Autodesk Fusion 360 part; units mm, degrees
sketch "Sketch1" plane through (0, 0, 0) normal (0, 0, 1) x (1, 0, 0)
  line L0 (-400.05, 260.35) -> (-387.35, 273.05)
  line L1 (-400.05, 12.7) -> (-387.35, 0)
  line L2 (-400.05, 260.35) -> (-400.05, 12.7)
  line L3 (0, 260.35) -> (-12.7, 273.05)
  line L4 (0, 12.7) -> (-12.7, 0)
  line L5 (0, 260.35) -> (0, 12.7)
  line L6 (-387.35, 0) -> (-12.7, 0)
  line L7 (-387.35, 273.05) -> (-12.7, 273.05)
  line L8 (-6.35, 257.7197) -> (-15.3303, 266.7)
  line L9 (-384.7197, 266.7) -> (-15.3303, 266.7)
  line L10 (-393.7, 257.7197) -> (-384.7197, 266.7)
  line L11 (-393.7, 257.7197) -> (-393.7, 15.3303)
  line L12 (-393.7, 15.3303) -> (-384.7197, 6.35)
  line L13 (-384.7197, 6.35) -> (-15.3303, 6.35)
  line L14 (-6.35, 15.3303) -> (-15.3303, 6.35)
  line L15 (-6.35, 257.7197) -> (-6.35, 15.3303)
  dimension "d5" = 6.35
extrude "Extrude1" add sketch "Sketch1" along normal blind 0.254 contours L0 L1 L2 L3 L4 L5 L6 L7 | L8 L9 L10 L11 L12 L13 L14 L15
extrude "Extrude2" add sketch "Sketch1" along normal blind 69.85
sketch "Sketch2" plane through (0, 0, 69.85) normal (0, 0, 1) x (-1, 0, 0)
  line L0 (393.7, -15.3303) -> (393.7, -257.7197)
  line L1 (393.7, -257.7197) -> (384.7197, -266.7)
  line L2 (384.7197, -266.7) -> (15.3303, -266.7)
  line L3 (15.3303, -266.7) -> (6.35, -257.7197)
  line L4 (6.35, -257.7197) -> (6.35, -15.3303)
  line L5 (6.35, -15.3303) -> (15.3303, -6.35)
  line L6 (15.3303, -6.35) -> (384.7197, -6.35)
  line L7 (384.7197, -6.35) -> (393.7, -15.3303)
  line L8 (400.05, -260.35) -> (400.05, -12.7)
  line L9 (400.05, -12.7) -> (387.35, 0)
  line L10 (387.35, 0) -> (12.7, 0)
  line L11 (12.7, 0) -> (0, -12.7)
  line L12 (0, -12.7) -> (0, -260.35)
  line L13 (0, -260.35) -> (12.7, -273.05)
  line L14 (12.7, -273.05) -> (387.35, -273.05)
  line L15 (387.35, -273.05) -> (400.05, -260.35)
  line L16 (393.7, -162.4342) -> (393.7, -166.61)
  line L17 (295.275, -266.7) -> (288.925, -266.7)
  line L18 (393.7, -193.675) -> (295.275, -193.675)
  line L19 (393.7, -193.675) -> (295.275, -193.675)
  line L20 (295.275, -193.675) -> (295.275, -187.325)
  line L21 (295.275, -187.325) -> (393.7, -187.325)
  line L22 (393.7, -187.325) -> (393.7, -193.675)
  line L23 (295.275, -187.325) -> (295.275, -193.675)
  line L24 (2.1633, -60.325) -> (288.925, -60.325)
  line L25 (288.925, -60.325) -> (288.925, -187.325)
  line L26 (2.1633, -60.325) -> (393.7, -60.325)
  line L27 (393.7, -60.325) -> (393.7, -53.975)
  line L28 (393.7, -53.975) -> (2.1633, -53.975)
  line L29 (2.1633, -53.975) -> (2.1633, -60.325)
  line L30 (295.275, -53.975) -> (288.925, -53.975)
  line L31 (288.925, -187.325) -> (123.825, -187.325)
  line L32 (123.825, -187.325) -> (117.475, -187.325)
  line L33 (117.475, -187.325) -> (123.825, -187.325)
  line L34 (123.825, -187.325) -> (123.825, -60.325)
  line L35 (123.825, -60.325) -> (117.475, -60.325)
  line L36 (117.475, -60.325) -> (117.475, -187.325)
  line L37 (295.275, -187.325) -> (288.925, -187.325)
  line L38 (288.925, -187.325) -> (288.925, -60.325)
  line L39 (288.925, -60.325) -> (295.275, -60.325)
  line L40 (295.275, -60.325) -> (295.275, -187.325)
  line L41 (295.275, -266.7) -> (288.925, -266.7)
  line L42 (288.925, -266.7) -> (288.925, -193.675)
  line L43 (288.925, -193.675) -> (295.275, -193.675)
  line L44 (295.275, -193.675) -> (295.275, -266.7)
  line L45 (117.475, -60.325) -> (123.825, -60.325)
  line L46 (123.825, -60.325) -> (123.825, -130.175)
  line L47 (123.825, -130.175) -> (117.475, -130.175)
  line L48 (117.475, -130.175) -> (117.475, -60.325)
  line L49 (117.475, -130.175) -> (6.35, -130.175)
  line L50 (6.35, -130.175) -> (6.35, -136.525)
  line L51 (6.35, -136.525) -> (117.475, -136.525)
  line L52 (117.475, -136.525) -> (117.475, -130.175)
  line L53 (117.475, -187.325) -> (393.7, -187.325)
  line L54 (393.7, -187.325) -> (393.7, -193.675)
  line L55 (393.7, -193.675) -> (117.475, -193.675)
  line L56 (117.475, -193.675) -> (117.475, -187.325)
  line L57 (123.825, -193.675) -> (117.475, -193.675)
  line L58 (117.475, -193.675) -> (117.475, -266.7)
  line L59 (117.475, -266.7) -> (123.825, -266.7)
  line L60 (123.825, -266.7) -> (123.825, -193.675)
  dimension "d11" = 6.35
  dimension "d12" = 73.025
  dimension "d13" = 6.35
  dimension "d15" = 6.35
  dimension "d17" = 6.35
  dimension "d18" = 165.1
  dimension "d19" = 6.35
  dimension "d22" = 127
  dimension "d23" = 6.35
  dimension "d24" = 69.85
  dimension "d25" = 6.35
extrude "Extrude3" add sketch "Sketch2" against normal blind 76.2 contours L0 L4 L24 L26 L27 L28 L30 L35 L39 L45 | L25 L26 L37 L38 L39 L40 L53 | L0 L18 L19 L20 L21 L22 L23 L53 L54 L55 | L20 L23 L31 L32 L33 L37 L43 L53 L55 L56 L57 | L4 L24 L26 L28 L29 | L24 L26 L34 L35 L36 L45 L46 L47 L48 | L2 L17 L41 L42 L43 L44 L55 | L32 L33 L34 L36 L47 L52 L53 | L4 L36 L49 L50 L51 L52 | L2 L55 L57 L58 L59 L60
The model under review builds one solid part; all positions refer to its coordinate system, in mm. Round coordinates to 2 decimals unless told otherwise and drop trailing zeros. Loops run counter-clockwise (first coordinate to the right, second up) from the corner with the lowest first, then second, coordinate; pieces in that order, holes last. Notation, with made-up numbers: (57, 24.25) -> (115, 24.25) arc R13 ccw to (115, 48.25) -> close; hole circle Ø3 at (54, 54.5). An arc over 180 degrees is marked (long way). Return JSON: item names as keys, results as strings.
(1) Add section D-D on y = 212.5. Write out the cut boundary in (x, z) (3 decimals).
Solved:
{"outline": "(-400.05, 0) -> (-295.275, 0) -> (-295.275, -6.35) -> (-288.925, -6.35) -> (-288.925, 0) -> (-123.825, 0) -> (-123.825, -6.35) -> (-117.475, -6.35) -> (-117.475, 0) -> (0, 0) -> (0, 69.85) -> (-6.35, 69.85) -> (-6.35, 0.254) -> (-117.475, 0.254) -> (-117.475, 69.85) -> (-123.825, 69.85) -> (-123.825, 0.254) -> (-288.925, 0.254) -> (-288.925, 69.85) -> (-295.275, 69.85) -> (-295.275, 0.254) -> (-393.7, 0.254) -> (-393.7, 69.85) -> (-400.05, 69.85) -> close"}
(2) For line 1 (X direction, y = 207, z = 18.5) (3 decimals); line 2 (Y direction, x = -149, z = 65) (3 decimals); line 3 (Y direction, x = -35, z = 64) (3 decimals), list the stretches that pass through material, from the lowest coordinate up.
Solved:
{"line 1": "-400.05 to -393.7, -295.275 to -288.925, -123.825 to -117.475, -6.35 to 0", "line 2": "0 to 6.35, 53.975 to 60.325, 187.325 to 193.675, 266.7 to 273.05", "line 3": "0 to 6.35, 53.975 to 60.325, 130.175 to 136.525, 266.7 to 273.05"}
(3) Add section B-B on x = -227. Write out the cut boundary in (y, z) (3 decimals), plus the area to 3 significant figures.
Solved:
{"outline": "(0, 0) -> (53.975, 0) -> (53.975, -6.35) -> (60.325, -6.35) -> (60.325, 0) -> (187.325, 0) -> (187.325, -6.35) -> (193.675, -6.35) -> (193.675, 0) -> (273.05, 0) -> (273.05, 69.85) -> (266.7, 69.85) -> (266.7, 0.254) -> (193.675, 0.254) -> (193.675, 69.85) -> (187.325, 69.85) -> (187.325, 0.254) -> (60.325, 0.254) -> (60.325, 69.85) -> (53.975, 69.85) -> (53.975, 0.254) -> (6.35, 0.254) -> (6.35, 69.85) -> (0, 69.85) -> close", "area": "1,920 mm2"}
(4) Add section C-C on z = 29.5. State how many separate pieces and enclosed holes the cut face has, plus the area to 3 significant figures.
Solved:
{"separate pieces": "1", "enclosed holes": "7", "area": "15,700 mm2"}
(5) The part is to be moulded in two halves that separate along X. For faces 1 (the flat face through (-197, 57, -6.35)), 2 (the flat face through (-123.825, 231, 36)), 3 (the flat face through (0, 138, 34)), 4 (the flat face through (-345, 193.675, 36)), say which applies: released by +X, released by -X, zero draft, split by the parting line, or undercut.
Solved:
{"face 1": "zero draft", "face 2": "undercut", "face 3": "released by +X", "face 4": "undercut"}
(6) For pin 1 (22 mm diameter, centred on x = -339, y = 242, fed in from +Z); pin 2 (7 mm diameter, centred on x = -218, z = -4.5, fed in from +Y) (3 decimals); pin 3 (3 mm diameter, centred on y = 114.5, z = -4.5, fed in from +X) (3 decimals), all flat-tipped, find the tip position at first contact; note any pin that passes through.
Solved:
{"pin 1": "z = 0.25", "pin 2": "y = 193.675", "pin 3": "x = -117.475"}
(7) Add section A-A on y = 32. Write out the cut boundary in (x, z), plus the area to 3 significant figures.
Solved:
{"outline": "(-400.05, 0) -> (0, 0) -> (0, 69.85) -> (-6.35, 69.85) -> (-6.35, 0.25) -> (-393.7, 0.25) -> (-393.7, 69.85) -> (-400.05, 69.85) -> close", "area": "985 mm2"}
